```python
from build123d import *

# Parameters (mm, degrees)
SKETCH1_W                = 20
SKETCH1_H                = 20
BOSS_EXTRUDE1_DEPTH      = 150
FILLET1_R                = 1
CUT_EXTRUDE1_DEPTH       = 151.665191733
F_5_0_5_DIAMETER_HOLE1_D = 5
FILLET2_R                = 2
FILLET3_R                = 0.5
FILLET4_R                = 0.5
FILLET5_R                = 0.5


with BuildPart() as part:
    # Sketch1 → Boss-Extrude1 (new body)
    with BuildSketch(Plane(origin=(0, 0, 0), x_dir=(0, 0, -1), z_dir=(1, 0, 0))):
        Rectangle(SKETCH1_W, SKETCH1_H)
    extrude(amount=BOSS_EXTRUDE1_DEPTH)

    # Fillet1
    fillet1_edges = [part.edges().sort_by_distance(p)[0] for p in [
        (75, 10, 10),
        (75, 10, -10),
        (75, -10, -10),
        (75, -10, 10),
    ]]
    fillet(fillet1_edges, radius=FILLET1_R)

    # Sketch3 → Cut-Extrude1 (cut, through all)
    with BuildSketch(Plane.ZY):
        Polygon((-3.6, 10), (3.6, 10), (3.6, 9.5), (3.1, 9.5), (3.1, 8.2), (5.63, 8.2), (5.63, 6.619949494), (2.910050506, 3.9), (-2.910050506, 3.9), (-5.63, 6.619949494), (-5.63, 8.2), (-3.1, 8.2), (-3.1, 9.5), (-3.6, 9.5), align=None)
        Polygon((10, 3.6), (10, -3.6), (9.5, -3.6), (9.5, -3.1), (8.2, -3.1), (8.2, -5.63), (6.619949494, -5.63), (3.9, -2.910050506), (3.9, 2.910050506), (6.619949494, 5.63), (8.2, 5.63), (8.2, 3.1), (9.5, 3.1), (9.5, 3.6), align=None)
        Polygon((3.6, -10), (-3.6, -10), (-3.6, -9.5), (-3.1, -9.5), (-3.1, -8.2), (-5.63, -8.2), (-5.63, -6.619949494), (-2.910050506, -3.9), (2.910050506, -3.9), (5.63, -6.619949494), (5.63, -8.2), (3.1, -8.2), (3.1, -9.5), (3.6, -9.5), align=None)
        Polygon((-10, -3.6), (-10, 3.6), (-9.5, 3.6), (-9.5, 3.1), (-8.2, 3.1), (-8.2, 5.63), (-6.619949494, 5.63), (-3.9, 2.910050506), (-3.9, -2.910050506), (-6.619949494, -5.63), (-8.2, -5.63), (-8.2, -3.1), (-9.5, -3.1), (-9.5, -3.6), align=None)
    extrude(amount=-CUT_EXTRUDE1_DEPTH, mode=Mode.SUBTRACT)

    # Ø5.0 (5) Diameter Hole1 (through all)
    with Locations(Plane.ZY):
        with Locations((0, 0)):
            Hole(F_5_0_5_DIAMETER_HOLE1_D / 2)

    # Fillet2
    fillet2_edges = [part.edges().sort_by_distance(p)[0] for p in [
        (75, -3.9, -2.910050506),
        (75, -3.9, 2.910050506),
        (75, 2.910050506, -3.9),
        (75, -2.910050506, -3.9),
        (75, -2.910050506, 3.9),
        (75, 2.910050506, 3.9),
        (75, 3.9, 2.910050506),
        (75, 3.9, -2.910050506),
    ]]
    fillet(fillet2_edges, radius=FILLET2_R)

    # Fillet3
    fillet3_edges = [part.edges().sort_by_distance(p)[0] for p in [
        (75, 3.6, -10),
        (75, 3.1, -9.5),
        (75, 3.1, -8.2),
        (75, 5.63, -8.2),
        (75, 5.63, -6.619949494),
        (75, 3.6, 10),
        (75, 3.1, 9.5),
        (75, 3.1, 8.2),
        (75, 5.63, 8.2),
        (75, 5.63, 6.619949494),
        (75, 6.619949494, 5.63),
        (75, 8.2, 5.63),
        (75, 8.2, 3.1),
        (75, 9.5, 3.1),
        (75, 10, 3.6),
        (75, 9.5, -3.1),
        (75, 10, -3.6),
        (75, 8.2, -3.1),
        (75, 8.2, -5.63),
        (75, 6.619949494, -5.63),
    ]]
    fillet(fillet3_edges, radius=FILLET3_R - 0.0001)  # a hair under: the kernel refuses the full size

    # Fillet4
    fillet4_edges = [part.edges().sort_by_distance(p)[0] for p in [
        (75, -3.6, 10),
        (75, -3.1, 9.5),
        (75, -3.1, 8.2),
        (75, -5.63, 8.2),
        (75, -5.63, 6.619949494),
        (75, -6.619949494, 5.63),
        (75, -8.2, 5.63),
        (75, -8.2, 3.1),
        (75, -10, 3.6),
        (75, -9.5, 3.1),
        (75, -10, -3.6),
        (75, -9.5, -3.1),
        (75, -8.2, -3.1),
        (75, -8.2, -5.63),
        (75, -6.619949494, -5.63),
        (75, -5.63, -6.619949494),
        (75, -5.63, -8.2),
        (75, -3.1, -8.2),
        (75, -3.1, -9.5),
        (75, -3.6, -10),
    ]]
    fillet(fillet4_edges, radius=FILLET4_R - 0.0001)  # a hair under: the kernel refuses the full size

    # Fillet5
    fillet5_edges = [part.edges().sort_by_distance(p)[0] for p in [
        (75, 3.6, 9.5),
        (75, 9.5, 3.6),
        (75, 9.5, -3.6),
        (75, 3.6, -9.5),
        (75, -3.6, 9.5),
        (75, -9.5, 3.6),
        (75, -9.5, -3.6),
        (75, -3.6, -9.5),
    ]]
    fillet(fillet5_edges, radius=FILLET5_R)


solid = part.part
```
Here's how the part is built. I have some questions about the finished solid (model axes, mm). A direction names the side the tool comes from. Give positions to 0.01 mm unless a question says otherwise; leave off trailing zeros. Write each loop counter-clockwise with the first axis right and the second up, starting at its lowest first coordinate (ties: lowest second). Pieces come first, ordered by that corner, then holes. Notation, with made-up numbers: (53, 38.25) -> (79, 38.25) arc R23 cw to (79, 72.25) -> close; hole circle Ø11 at (5.5, -39). An arc over 180 degrees is marked (long way). Write each question's results on one line, items separated by ' | '.
Item 1: If I drill on L1, parallel to Y at x = 140.5, z = -6.75; L2, parallel to Y at x = 120, z = 0; L3, parallel to Z at x = 42, y = -9, over which ranges is the centre line in solid material (lowest first)?
Output:
L1: y = -10 to -5.62, 5.62 to 10 | L2: y = -3.9 to -2.5, 2.5 to 3.9 | L3: z = -10 to -3.1, 3.1 to 10
Item 2: We'd pull the mould along Y, two halves only. Please class faces 4 (the face through (74, -3.9, 0)), 5 (the face through (74, -7, -10)), 6 (the face through (74, 0, 3.9)): pulls with the +Y half, pulls with the -Y half, needs draft (parallel to the pull), parting line crosses it, or undercut.
Output:
face 4: pulls with the -Y half | face 5: needs draft | face 6: undercut
Item 3: For pin 1 Ø3 at (y, z) = (0, 0) entering from -X; pin 2 Ø4.5 at (x, y) = (81, -0.5) entering from +Z (3 decimals); pin 3 Ø3.5 at (x, y) = (37.5, -0.5) entering from -Z, each with a flat end and sliding along its axis, tell me the tip position at first contact or that it passes through.
Output:
pin 1: passes through | pin 2: stops at z = 4.015 | pin 3: stops at z = -3.91
Item 4: On a 3-axis mill with a long thin cutter (end or side, diameter ignored), from which of +Z, -Z, +X, -X, +Y, -Y can I reach the whole of each face in a straight line? I mean faces 1 (the face through (74, 10, -7)), 2 (the face through (74, 3.9, 0)), 3 (the face through (74, 0, -3.9)). Say none if no direction works.
Output:
face 1: +Z, -Z, +X, -X, +Y | face 2: +X, -X, +Y | face 3: -Z, +X, -X
Item 5: Suppose I cut it at A-A on z = 0. Write out the boundary of the cut face in (x, y), plus the area to 3 significant figures.
Output:
outline: (0, -3.9) -> (150, -3.9) -> (150, -2.5) -> (0, -2.5) -> close; (0, 2.5) -> (150, 2.5) -> (150, 3.9) -> (0, 3.9) -> close | area: 420 mm^2
